from build123d import *

# Parameters (mm, degrees)
SKETCH1_W           = 38.1
SKETCH1_H           = 38.1
SKETCH1_R           = 9.525
BOSS_EXTRUDE1_DEPTH = 44.45
SKETCH2_R           = 6.858
CUT_EXTRUDE1_DEPTH  = 62.565534189
SKETCH3_R           = 5.55625
CUT_EXTRUDE2_DEPTH  = 19.05
SKETCH4_R           = 6.858
CUT_EXTRUDE3_DEPTH  = 19.05


with BuildPart() as part:
    # Sketch1 → Boss-Extrude1 (new, symmetric)
    with BuildSketch(Plane.XY):
        Rectangle(SKETCH1_W, SKETCH1_H)
        Circle(SKETCH1_R, mode=Mode.SUBTRACT)
    extrude(amount=BOSS_EXTRUDE1_DEPTH, both=True)

    # Sketch2 → Cut-Extrude1 (cut, through all)
    with BuildSketch(Plane(origin=(19.05, 0, 0), x_dir=(0, 0, -1), z_dir=(1, 0, 0))):
        with Locations(Location((-15.875, 0, 0), (0, 0, 90))):
            Circle(SKETCH2_R)
    extrude(amount=-CUT_EXTRUDE1_DEPTH, mode=Mode.SUBTRACT)

    # Sketch3 → Cut-Extrude2 (cut)
    with BuildSketch(Plane(origin=(19.05, 0, 0), x_dir=(0, 0, -1), z_dir=(1, 0, 0))):
        with Locations(Location((15.875, 0, 0), (0, 0, 90))):
            Circle(SKETCH3_R)
    extrude(amount=-CUT_EXTRUDE2_DEPTH, mode=Mode.SUBTRACT)

    # Sketch4 → Cut-Extrude3 (cut)
    with BuildSketch(Plane.ZY.offset(19.05)):
        with Locations(Location((-15.875, 0, 0), (0, 0, 270))):
            Circle(SKETCH4_R)
    extrude(amount=-CUT_EXTRUDE3_DEPTH, mode=Mode.SUBTRACT)


solid = part.part
The listing builds one solid part. Answer for the finished solid, in the listing's coordinates (mm). Give positions to 0.01 mm unless a question says otherwise; leave off trailing zeros. Write each loop counter-clockwise with the first axis right and the second up, starting at its lowest first coordinate (ties: lowest second). Pieces come first, ordered by that corner, then holes.
1) Find the intervals of material crossed by L1, parallel to Z at x = -10.5, y = 0; L2, parallel to Z at x = 15.5, y = 0; L3, parallel to X at y = 0, z = 1 (3 decimals), in increasing order.
2) Section C-C (z = -34) is taken. Write down the section's boundary in (x, y) (3 decimals), and give its area (3 significant figures).
3) Section A-A (y = 0) is taken. Write down the section's boundary in (x, z) (3 decimals), and give its area (3 significant figures).
4) For a pull along Z with two mould halves and no side action, classify faces 1 (the face through (14.299, 6.335, 13.248)), 2 (the face through (-19.05, 0, 1)), 3 (the face through (-14.299, -6.541, -13.815)), 4 (the face through (-5, 9, -44.45)) as pulls with the +Z half, pulls with the -Z half, needs draft (parallel to the pull), parting line crosses it, or undercut.
5) Given P1, Ø10, axis at y = 0, z = -15.875, coming from the -X side, flat-ended and moving along its own axis, determine where the tip first touches the part or whether it passes through.
6) Section B-B (x = 0) is taken. Write down the section's boundary in (y, z) (3 decimals).
7) Section D-D (x = 15) is taken. Count the separate pieces of the cut face and the enclosed holes in it, and give its area (3 significant figures).
Response:
1. L1: z = -44.45 to -22.73, -9.02 to 9.02, 22.73 to 44.45
1. L2: z = -44.45 to -21.43, -10.32 to 9.02, 22.73 to 44.45
1. L3: x = -19.05 to -9.525, 9.525 to 19.05
2. outline: (-19.05, -19.05) - (19.05, -19.05) - (19.05, 19.05) - (-19.05, 19.05) - close; hole circle Ø19.05 at (0, 0)
2. area: 1,170 mm2
3. outline: (-19.05, -44.45) - (-9.525, -44.45) - (-9.525, -22.733) - (-19.05, -22.733) - close; (-19.05, -9.017) - (-9.525, -9.017) - (-9.525, 9.017) - (-19.05, 9.017) - close; (-19.05, 22.733) - (-9.525, 22.733) - (-9.525, 44.45) - (-19.05, 44.45) - close; (9.525, -44.45) - (19.05, -44.45) - (19.05, -21.431) - (9.525, -21.431) - close; (9.525, -10.319) - (19.05, -10.319) - (19.05, 9.017) - (9.525, 9.017) - close; (9.525, 22.733) - (19.05, 22.733) - (19.05, 44.45) - (9.525, 44.45) - close
3. area: 1,200 mm2
4. face 1: undercut
4. face 2: needs draft
4. face 3: undercut
4. face 4: pulls with the -Z half
5. P1: passes through
6. outline: (-19.05, -44.45) - (-9.525, -44.45) - (-9.525, 44.45) - (-19.05, 44.45) - close; (9.525, -44.45) - (19.05, -44.45) - (19.05, 44.45) - (9.525, 44.45) - close
7. separate pieces: 1
7. enclosed holes: 2
7. area: 3,140 mm2
